from build123d import *

# Parameters (mm, degrees)
SKETCH1_R           = 10
BOSS_EXTRUDE1_DEPTH = 15


with BuildPart() as part:
    # Sketch1 (on Front Plane) → Boss-Extrude1 (new body)
    with BuildSketch(Plane.XY):
        Polygon((-70, 19.808892587), (-70, -40.191107413), (70, -40.191107413), (70, 9.808892587), (50, 9.808892587), (50, 69.808892587), (20, 69.808892587), (20, 39.808892587), (-20, 39.808892587), (-20, 69.808892587), (-50, 69.808892587), (-50, 19.808892587), align=None)
        with Locations((-45, -20.191107413)):
            Circle(SKETCH1_R, mode=Mode.SUBTRACT)
        with Locations((0, -20.191107413)):
            Circle(SKETCH1_R, mode=Mode.SUBTRACT)
        with Locations((45, -20.191107413)):
            Circle(SKETCH1_R, mode=Mode.SUBTRACT)
    extrude(amount=BOSS_EXTRUDE1_DEPTH)


solid = part.part
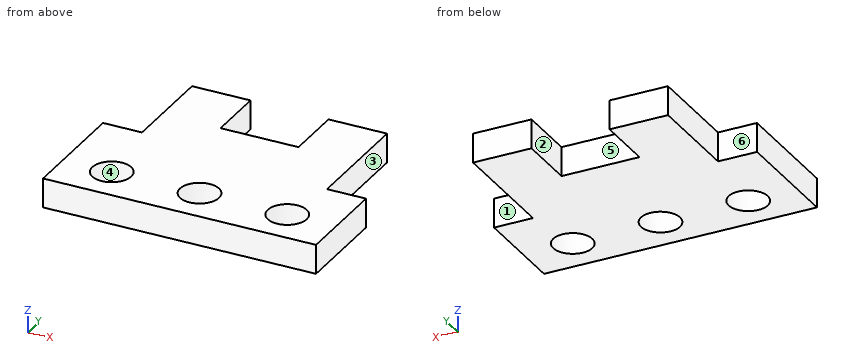
The model under review builds one solid part; all positions refer to its coordinate system, in mm. Face numbers are marked on the shaded views. A direction names the side the tool comes from. Round coordinates to 2 decimals unless told otherwise and drop trailing zeros. Loops run counter-clockwise (first coordinate to the right, second up) from the corner with the lowest first, then second, coordinate; pieces in that order, holes last. Notation, with made-up numbers: M 86.25,19.25 L 114.25,19.25 A9 cw 114.25,23.25 Z; hole C 83,-23 d5. An arc over 180 degrees is marked long. Answer as a JSON object with one key per item and string values.
Item 1: We need section B-B, the plane y = 61. State the section outline as (x, z) points, and give its area (3 significant figures).
Check sheet entries:
{"outline": "M -50,0 L -20,0 L -20,15 L -50,15 Z; M 20,0 L 50,0 L 50,15 L 20,15 Z", "area": "900 mm2"}
Item 2: We need section D-D, the plane z = 3.25. State the section outline as (x, y) points.
Check sheet entries:
{"outline": "M -70,-40.19 L 70,-40.19 L 70,9.81 L 50,9.81 L 50,69.81 L 20,69.81 L 20,39.81 L -20,39.81 L -20,69.81 L -50,69.81 L -50,19.81 L -70,19.81 Z; hole C -45,-20.19 d20; hole C 0,-20.19 d20; hole C 45,-20.19 d20"}
Item 3: The part is to be moulded in two halves that separate along X. For the marked faces 1, 2 and 3, say which applies: +X half, -X half, draft (parallel to the pull), parting line (faces both ways), or undercut.
Check sheet entries:
{"face 1": "draft", "face 2": "undercut", "face 3": "+X half"}
Item 4: For line 1 along X through (y, z) = (-21, 7.5); line 2 along Y through (x, z) = (45, 11.5); line 3 along Y through (x, z) = (0, 7.5), list the stretches that pass through material, from the lowest coordinate up.
Check sheet entries:
{"line 1": "-70 to -54.97, -35.03 to -9.97, 9.97 to 35.03, 54.97 to 70", "line 2": "-40.19 to -30.19, -10.19 to 69.81", "line 3": "-40.19 to -30.19, -10.19 to 39.81"}
Item 5: We need section A-A, the plane x = -45. State the section outline as (y, z) points, and give its area (3 significant figures).
Check sheet entries:
{"outline": "M -40.19,0 L -30.19,0 L -30.19,15 L -40.19,15 Z; M -10.19,0 L 69.81,0 L 69.81,15 L -10.19,15 Z", "area": "1,350 mm2"}
Item 6: Tool access review of the marked faces 4, 5 and 6: name each direction out of +Z, -Z, +X, -X, +Y, -Y from which nothing blocks a thin tool from reaching the whole face with its end or side.
Check sheet entries:
{"face 4": "+Z, -Z", "face 5": "+Z, -Z, +Y", "face 6": "+Z, -Z, -X, +Y"}
Item 7: We need section C-C, the plane y = -17. State the section outline as (x, z) points, and give its area (3 significant figures).
Check sheet entries:
{"outline": "M -70,0 L -54.48,0 L -54.48,15 L -70,15 Z; M -35.52,0 L -9.48,0 L -9.48,15 L -35.52,15 Z; M 9.48,0 L 35.52,0 L 35.52,15 L 9.48,15 Z; M 54.48,0 L 70,0 L 70,15 L 54.48,15 Z", "area": "1,250 mm2"}
Item 8: Clearance check with flat-ended pins moving along their axes: P1, Ø6, axis at y = 29, z = 2, coming from the +X side; P2, Ø4.5, axis at x = -62, z = 4.5, coming from the +Y side; P3, Ø7.5, axis at x = -0.5, z = 5.5, coming from the +Y side. State where each tip first meets the part, or that it passes through.
Check sheet entries:
{"P1": "x = 50", "P2": "y = 19.81", "P3": "y = 39.81"}
